The drawing under review shows one solid part. Ordinate dimensions are in mm from its lowest x, y, z. Coordinates: 2 decimals unless noted, no trailing zeros. Write each loop counter-clockwise with the first axis right and the second up, starting at its lowest first coordinate (ties: lowest second). Pieces come first, ordered by that corner, then holes. Notation, with made-up numbers: M 16.5,67 L 44.5,67 A13 cw 44.5,84 Z; hole C 59,38 d2. An arc over 180 degrees is marked long. Write item = value, one per line.
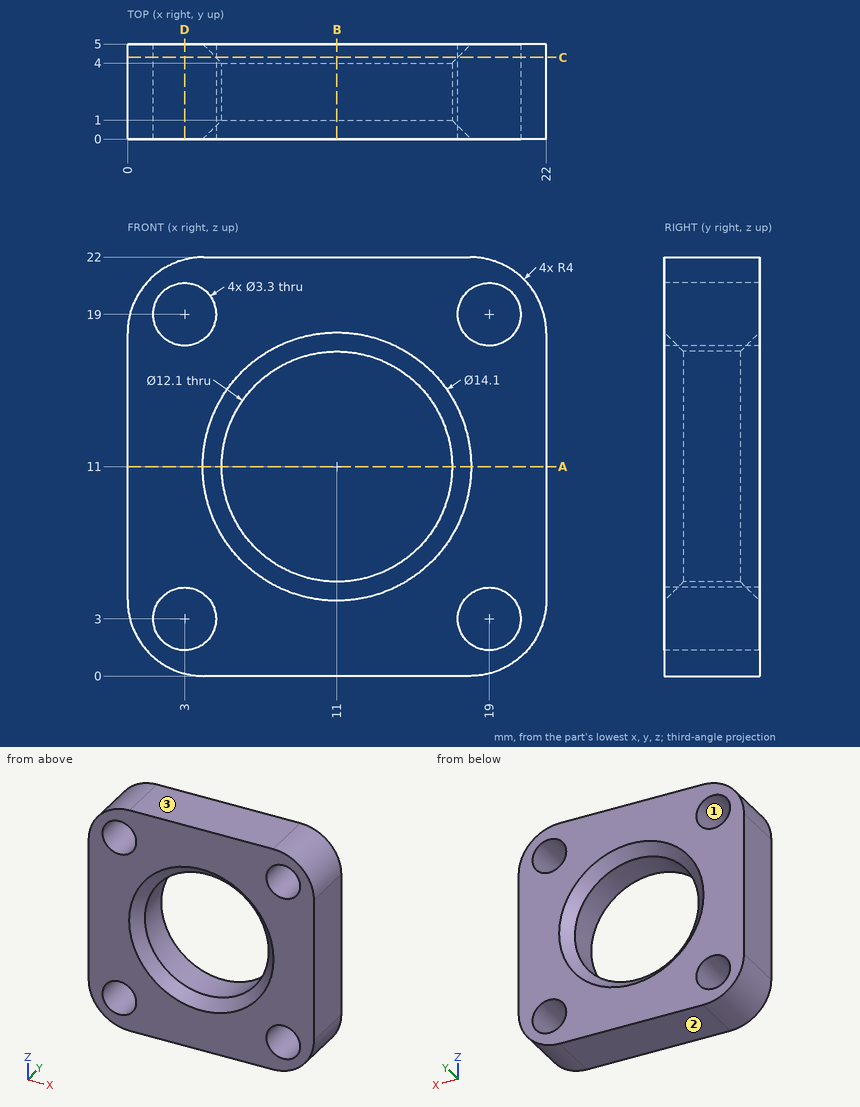
Q1. For P1, Ø5.5, axis at x = 19, z = 19, coming from the +Y side, flat-tipped, find the tip position at first contact; note if it passes through.
Check result:
P1 = 5
Q2. Wall thickness on line 1 (Z direction, x = 19, y = 2.35); line 2 (X direction, y = 4.05, z = 20.25); line 3 (Z direction, x = 19.75, y = 4.25): over which ranges is each line inside the solid? List them lowest first.
Check result:
line_1 = 0.13 to 1.35, 4.65 to 17.35, 20.65 to 21.87
line_2 = 0.69 to 1.92, 4.08 to 17.92, 20.08 to 21.31
line_3 = 0.4 to 1.53, 4.47 to 17.53, 20.47 to 21.6
Q3. Consider section C-C, the plane y = 4.3. State the section outline as (x, z) points, and give its area (3 significant figures).
Check result:
outline = M 0,4 A4 ccw 4,0 L 18,0 A4 ccw 22,4 L 22,18 A4 ccw 18,22 L 4,22 A4 ccw 0,18 Z; hole C 3,3 d3.3; hole C 3,19 d3.3; hole C 11,11 d12.7; hole C 19,3 d3.3; hole C 19,19 d3.3
area = 309 mm²
Q4. Consider section B-B, the plane x = 11. State the section outline as (y, z) points, and give its area (3 significant figures).
Check result:
outline = M 0,0 L 5,0 L 5,3.95 L 4,4.95 L 1,4.95 L 0,3.95 Z; M 0,18.05 L 1,17.05 L 4,17.05 L 5,18.05 L 5,22 L 0,22 Z
area = 47.5 mm²
Q5. Consider section A-A, the plane z = 11. State the section outline as (x, y) points.
Check result:
outline = M 0,0 L 3.95,0 L 4.95,1 L 4.95,4 L 3.95,5 L 0,5 Z; M 17.05,1 L 18.05,0 L 22,0 L 22,5 L 18.05,5 L 17.05,4 Z
Q6. Consider section D-D, the plane x = 3. State the section outline as (y, z) points.
Check result:
outline = M 0,0.13 L 5,0.13 L 5,1.35 L 0,1.35 Z; M 0,4.65 L 5,4.65 L 5,17.35 L 0,17.35 Z; M 0,20.65 L 5,20.65 L 5,21.87 L 0,21.87 Z
Q7. The part is to be moulded in two halves that separate along Z. For the marked faces 1, 2 and 3, say which applies: +Z half, -Z half, draft (parallel to the pull), parting line (faces both ways), or undercut.
Check result:
face_1 = undercut
face_2 = -Z half
face_3 = +Z half
